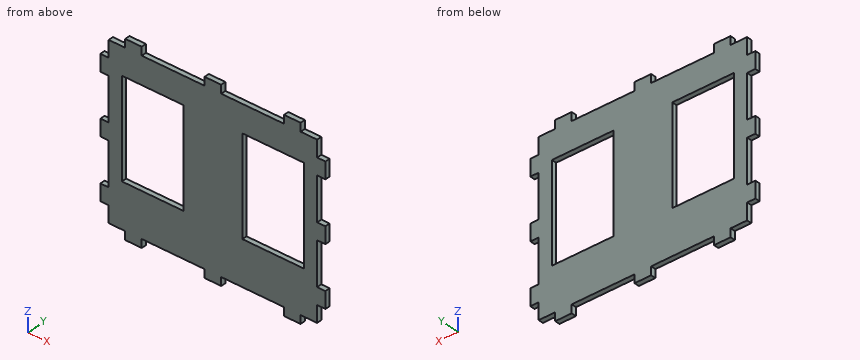
```python
from build123d import *

# Parameters (mm, degrees)
F0_W     = 6.35
F0_H     = 12.7
F0_W_2   = 47.2488999367
F0_H_2   = 75
F0_W_3   = 12.7
F0_H_3   = 6.35
F1_DEPTH = 3.81


# Not quite as in the source:
# - a feature names something its author has since deleted; it is built from what else it names


with BuildPart() as f1:
    # F0 (on Front) → F1 (new body)
    with BuildSketch(Plane.XZ):
        with Locations((-354.6769669852, 49.3793434303)):
            Rectangle(F0_W, F0_H)
        with Locations((-361.0269669852, 49.3793434303)):
            Rectangle(F0_W, F0_H)
        Polygon((-332.4519669852, -61.5706565697), (-284.2019669852, -61.5706565697), (-284.2019669852, -55.2206565697), (-277.8519669852, -55.2206565697), (-277.8519669852, 62.0793434303), (-284.2019669852, 62.0793434303), (-284.2019669852, 68.4293434303), (-332.4519669852, 68.4293434303), (-332.4519669852, 62.0793434303), (-345.1519669852, 62.0793434303), (-345.1519669852, 68.4293434303), (-357.8519669852, 68.4293434303), (-357.8519669852, 55.7293434303), (-351.5019669852, 55.7293434303), (-351.5019669852, 43.0293434303), (-357.8519669852, 43.0293434303), (-357.8519669852, 9.7793434303), (-351.5019669852, 9.7793434303), (-351.5019669852, -2.9206565697), (-357.8519669852, -2.9206565697), (-357.8519669852, -36.1706565697), (-351.5019669852, -36.1706565697), (-351.5019669852, -48.8706565697), (-357.8519669852, -48.8706565697), (-357.8519669852, -61.5706565697), (-345.1519669852, -61.5706565697), (-345.1519669852, -55.2206565697), (-332.4519669852, -55.2206565697), align=None)
        with Locations((-324.0675170169, 10.0176490168)):
            Rectangle(F0_W_2, F0_H_2, mode=Mode.SUBTRACT)
        with Locations((-338.8019669852, 65.2543434303)):
            Rectangle(F0_W_3, F0_H_3)
        with Locations((-338.8019669852, 71.6043434303)):
            Rectangle(F0_W_3, F0_H_3)
        Polygon((-210.5519669852, -61.5706565697), (-197.8519669852, -61.5706565697), (-197.8519669852, -48.8706565697), (-204.2019669852, -48.8706565697), (-204.2019669852, -36.1706565697), (-197.8519669852, -36.1706565697), (-197.8519669852, -2.9206565697), (-204.2019669852, -2.9206565697), (-204.2019669852, 9.7793434303), (-197.8519669852, 9.7793434303), (-197.8519669852, 43.0293434303), (-204.2019669852, 43.0293434303), (-204.2019669852, 55.7293434303), (-197.8519669852, 55.7293434303), (-197.8519669852, 68.4293434303), (-210.5519669852, 68.4293434303), (-210.5519669852, 62.0793434303), (-223.2519669852, 62.0793434303), (-223.2519669852, 68.4293434303), (-271.5019669852, 68.4293434303), (-271.5019669852, 62.0793434303), (-277.8519669852, 62.0793434303), (-277.8519669852, -55.2206565697), (-271.5019669852, -55.2206565697), (-271.5019669852, -61.5706565697), (-223.2519669852, -61.5706565697), (-223.2519669852, -55.2206565697), (-210.5519669852, -55.2206565697), align=None)
        with Locations((-231.6364169536, 10.0176490168)):
            Rectangle(F0_W_2, F0_H_2, mode=Mode.SUBTRACT)
        Polygon((-284.2019669852, 68.4293434303), (-277.8519669852, 68.4293434303), (-271.5019669852, 68.4293434303), (-271.5019669852, 74.7793434303), (-284.2019669852, 74.7793434303), align=None)
        with Locations((-274.6769669852, 65.2543434303)):
            Rectangle(F0_W, F0_H_3)
        with Locations((-281.0269669852, 65.2543434303)):
            Rectangle(F0_W, F0_H_3)
        with Locations((-216.9019669852, 71.6043434303)):
            Rectangle(F0_W_3, F0_H_3)
        with Locations((-216.9019669852, 65.2543434303)):
            Rectangle(F0_W_3, F0_H_3)
        with Locations((-354.6769669852, 3.4293434303)):
            Rectangle(F0_W, F0_H)
        with Locations((-361.0269669852, 3.4293434303)):
            Rectangle(F0_W, F0_H)
        with Locations((-361.0269669852, -42.5206565697)):
            Rectangle(F0_W, F0_H)
        with Locations((-338.8019669852, -64.7456565697)):
            Rectangle(F0_W_3, F0_H_3)
        with Locations((-354.6769669852, -42.5206565697)):
            Rectangle(F0_W, F0_H)
        with Locations((-338.8019669852, -58.3956565697)):
            Rectangle(F0_W_3, F0_H_3)
        with Locations((-281.0269669852, -58.3956565697)):
            Rectangle(F0_W, F0_H_3)
        with Locations((-274.6769669852, -58.3956565697)):
            Rectangle(F0_W, F0_H_3)
        Polygon((-271.5019669852, -67.9206565697), (-271.5019669852, -61.5706565697), (-277.8519669852, -61.5706565697), (-284.2019669852, -61.5706565697), (-284.2019669852, -67.9206565697), align=None)
        with Locations((-216.9019669852, -64.7456565697)):
            Rectangle(F0_W_3, F0_H_3)
        with Locations((-216.9019669852, -58.3956565697)):
            Rectangle(F0_W_3, F0_H_3)
        with Locations((-201.0269669852, -42.5206565697)):
            Rectangle(F0_W, F0_H)
        with Locations((-194.6769669852, -42.5206565697)):
            Rectangle(F0_W, F0_H)
        with Locations((-201.0269669852, 3.4293434303)):
            Rectangle(F0_W, F0_H)
        with Locations((-194.6769669852, 3.4293434303)):
            Rectangle(F0_W, F0_H)
        with Locations((-201.0269669852, 49.3793434303)):
            Rectangle(F0_W, F0_H)
        with Locations((-194.6769669852, 49.3793434303)):
            Rectangle(F0_W, F0_H)
    extrude(amount=F1_DEPTH)


solid = f1.part
```
The model under review builds one solid part; all positions refer to its coordinate system, in mm. Coordinates: 2 decimals unless noted, no trailing zeros. Write each loop counter-clockwise with the first axis right and the second up, starting at its lowest first coordinate (ties: lowest second). Pieces come first, ordered by that corner, then holes. Notation, with made-up numbers: (56.25, 75.25) - (104.25, 75.25) arc R23 ccw to (104.25, 104.25) - close; hole circle Ø6 at (7, 53). An arc over 180 degrees is marked (long way). Answer in a Markdown table with one row per item. Add a question column.
Q1. Consider section B-B on x = -322. Give the boundary of the cut face in (y, z), then the cut area to 3 significant figures.
Q2. Consider section D-D on y = -1.9. Give the number of separate pieces and of enclosed holes in the cut face, then the cut area to 3 significant figures.
Q3. To check wall thickness, follow line 1 along X through (y, z) = (-1.25, 3); line 2 along X through (y, z) = (-3, -7); line 3 along Z through (x, y) = (-306.5, -2.3). State the ranges of each line that lie inside material, in increasing order. Write a range as from..to.
Q4. Clearance check with flat-ended pins moving along their axes: pin 1 (1.9 mm diameter, centred on y = -1.5, z = -65.5, fed in from -X); pin 2 (1.9 mm diameter, centred on x = -348.5, y = -1.5, fed in from +Z); pin 3 (10 mm diameter, centred on x = -282, z = 5.5, fed in from +Y); pin 4 (1.9 mm diameter, centred on y = -2, z = -63.5, fed in from +X). State where each tip first meets the part, or that it passes through.
Q5. Consider section C-C on z = 38.5. Give the boundary of the cut face in (x, y), then the cut area to 3 significant figures.
Q6. Consider section A-A on z = -0.5. Give the boundary of the cut face in (x, y).
Answers below:
| question | item | result |
|---|---|---|
| 1 | outline | (-3.81, -61.57) - (0, -61.57) - (0, -27.48) - (-3.81, -27.48) - close; (-3.81, 47.52) - (0, 47.52) - (0, 68.43) - (-3.81, 68.43) - close |
| 1 | area | 210 mm² |
| 2 | separate pieces | 1 |
| 2 | enclosed holes | 2 |
| 2 | area | 14,700 mm² |
| 3 | line 1 | -364.2..-347.69, -300.44..-255.26, -208.01..-191.5 |
| 3 | line 2 | -357.85..-347.69, -300.44..-255.26, -208.01..-197.85 |
| 3 | line 3 | -61.57..-27.48, 47.52..68.43 |
| 4 | pin 1 | x = -345.15 |
| 4 | pin 2 | z = 68.43 |
| 4 | pin 3 | y = 0 |
| 4 | pin 4 | x = -210.55 |
| 5 | outline | (-357.85, -3.81) - (-347.69, -3.81) - (-347.69, 0) - (-357.85, 0) - close; (-300.44, -3.81) - (-255.26, -3.81) - (-255.26, 0) - (-300.44, 0) - close; (-208.01, -3.81) - (-197.85, -3.81) - (-197.85, 0) - (-208.01, 0) - close |
| 5 | area | 250 mm² |
| 6 | outline | (-364.2, -3.81) - (-347.69, -3.81) - (-347.69, 0) - (-364.2, 0) - close; (-300.44, -3.81) - (-255.26, -3.81) - (-255.26, 0) - (-300.44, 0) - close; (-208.01, -3.81) - (-191.5, -3.81) - (-191.5, 0) - (-208.01, 0) - close |
